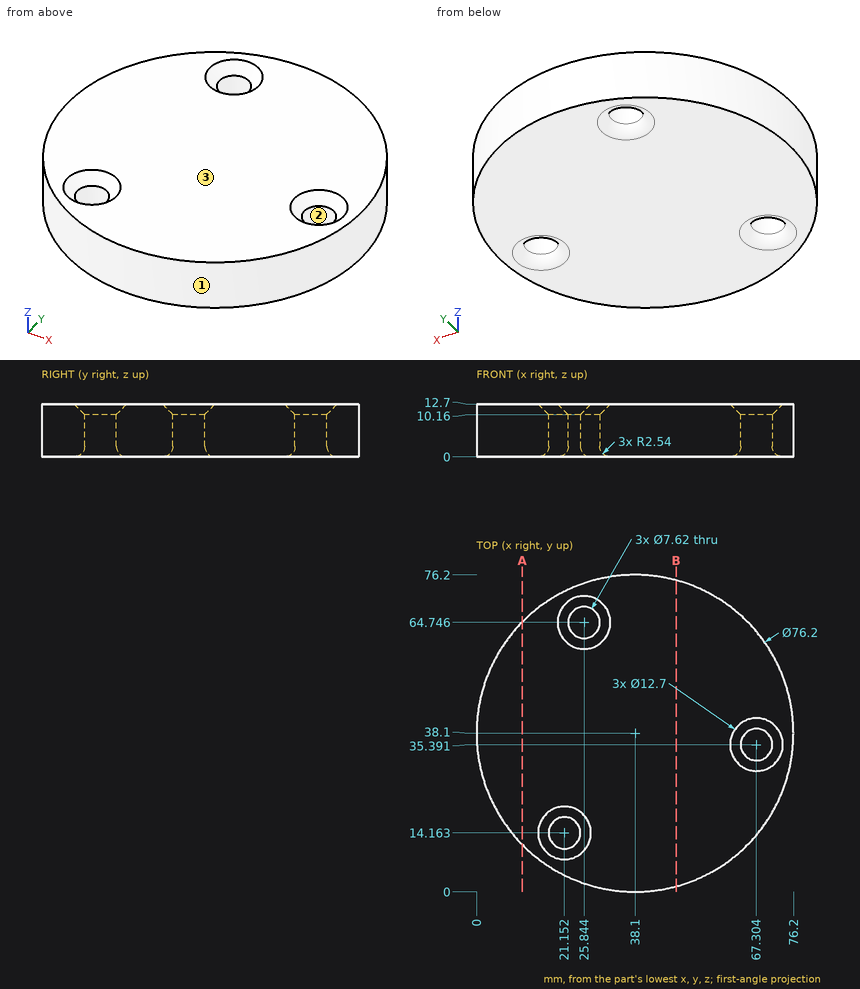
Study the drawing (mm; zero at the part's minimum x, y, z) and answer. Round coordinates to 2 decimals unless told otherwise and drop trailing zeros. Order: outer loops, then holes, each group sorted by start corner. A loop starts at its lowest first (then second) coordinate and runs counter-clockwise, first axis right, second up. Notation, with made-up numbers: (20.5, 51.5) -> (29.5, 51.5) arc R12 ccw to (29.5, 63.5) -> close; hole circle Ø9 at (83.25, 20). An arc over 180 degrees is marked (long way). Write each question's results on one line, items separated by ' | '. Start each with the question number.
Q1. Find section B-B (x = 48). Determine the outline of the cut face in (y, z), then the cut area to 4 significant figures.
Q2. Straight lines are drawn through the part: probe 1 along Y at (x, z) = (25.5, 12.25) (1 decimal); probe 2 along Y at (x, z) = (25.5, 6); probe 3 along Y at (x, z) = (68, 7) (1 decimal). For each, find the intervals that lie inside material, in ascending order. Write a range as from..to.
Q3. Each of these flat-tipped pins is pushed along its axis until it touches: pin 1 (9 mm diameter, centred on x = 67.3, y = 35.39, fed in from -Z) (1 decimal); pin 2 (12 mm diameter, centred on x = 21.15, y = 14.16, fed in from -Z); pin 3 (3 mm diameter, centred on x = 32.5, z = 7, fed in from +Y); pin 4 (6 mm diameter, centred on x = 25.84, y = 64.75, fed in from +Z). Where does it stop, or does it pass through?
Q4. The mould has two halves that part along Y. Classify the marked faces 1, 2 and 3: pulls with the +Y half, pulls with the -Y half, needs draft (parallel to the pull), parting line crosses it, or undercut.
Q5. Find section A-A (x = 11). Determine the outline of the cut face in (y, z).
Worked answers:
1) outline: (1.31, 0) -> (74.89, 0) -> (74.89, 12.7) -> (1.31, 12.7) -> close | area: 934.5 mm2
2) probe 1: y = 2.1..10.2, 18.2..58.9, 70.6..74.1 | probe 2: y = 2.14..60.95, 68.54..74.06 | probe 3: y = 14.5..31.6, 39.1..61.7
3) pin 1: stops at z = 0.8 | pin 2: stops at z = 0.02 | pin 3: stops at y = 75.98 | pin 4: passes through
4) face 1: parting line crosses it | face 2: undercut | face 3: needs draft
5) outline: (11.32, 0) -> (64.88, 0) -> (64.88, 12.7) -> (11.32, 12.7) -> close
